The listing builds one solid part. Answer for the finished solid, in the listing's coordinates (mm). A direction names the side the tool comes from. Give positions to 0.01 mm unless a question says otherwise; leave off trailing zeros. Order: outer loops, then holes, each group sorted by start corner. A loop starts at its lowest first (then second) coordinate and runs counter-clockwise, first axis right, second up.
```python
from build123d import *

# Parameters (mm, degrees)
EXTRUDE_THIN1_DEPTH      = 100
F_4_0_4_DIAMETER_HOLE1_D = 4
FILLET3_R                = 5
FILLET2_R                = 1.5


with BuildPart() as part:
    # Sketch1 → Extrude-Thin1 (new body, symmetric)
    with BuildSketch(Plane(origin=(0, 0, 0), x_dir=(0, 0, -1), z_dir=(1, 0, 0))):
        Polygon((12.7, 40), (12.7, 0), (0, 0), (-12.7, 0), (-12.7, 20), (-17.7, 20), (-17.7, -5), (0, -5), (17.7, -5), (17.7, 40), align=None)
    extrude(amount=EXTRUDE_THIN1_DEPTH, both=True)

    # Ø4.0 (4) Diameter Hole1 (through all)
    with Locations(Plane(origin=(0, 13.65, 13.65), x_dir=(-1, 0, 0), z_dir=(0, 0.707106781, 0.707106781))):
        with Locations((80, -29.264527369), (-80, -29.264527369), (0, -29.264527369)):
            Hole(F_4_0_4_DIAMETER_HOLE1_D / 2)

    # Fillet3
    fillet3_edges = [part.edges().sort_by_distance(p)[0] for p in [
        (0, 0, -12.7),
    ]]
    fillet(fillet3_edges, radius=FILLET3_R)

    # Fillet2
    fillet2_edges = [part.edges().sort_by_distance(p)[0] for p in [
        (-100, 10, 12.7),
        (-100, 0, 2.5),
        (-100, 40, -15.2),
        (0, 20, 17.7),
        (0, 20, 12.7),
        (0, 0, 12.7),
        (0, 40, -12.7),
        (0, 40, -17.7),
        (100, 0, 2.5),
        (100, 10, 12.7),
        (100, 20, 15.2),
        (100, 7.5, 17.7),
        (-100, 22.5, -12.7),
        (100, 22.5, -12.7),
        (-100, 1.464466094, -11.235533906),
        (100, 1.464466094, -11.235533906),
        (100, 40, -15.2),
        (-100, 7.5, 17.7),
        (-100, 20, 15.2),
    ]]
    fillet(fillet2_edges, radius=FILLET2_R)


solid = part.part
```
1) Straight lines are drawn through the part: probe 1 along Z at (x, y) = (18, 14); probe 2 along Y at (x, z) = (8, 11); probe 3 along Y at (x, z) = (28.5, -14). For each, find the intervals that lie inside material, in ascending order.
Geometry says:
probe 1: z = -17.7 to -12.7, 12.7 to 17.7
probe 2: y = -5 to 0
probe 3: y = -5 to 39.99
2) Given P1, Ø5.5, axis at x = 19, z = 6, coming from the +Y side; P2, Ø8, axis at y = 3.5, z = -2, coming from the -X side; P3, Ø0.6, axis at x = -46.5, z = 15, coming from the +Y side; P4, Ø3, axis at y = 11, z = 10.5, coming from the +X side, each flat-ended and moving along its own axis, determine where each tip first touches the part or whether it passes through.
Geometry says:
P1: stops at y = 0
P2: stops at x = -99.62
P3: stops at y = 20
P4: passes through
3) A tool of negligible diameter and unlimited length cuts with its end or side. For faces 4 (the flat face through (1, 0, 2)), 5 (the cylindrical face through (-78.1, 25.7, -14.8)), from which of +Z, -Z, +X, -X, +Y, -Y can it reach the whole face along a straight path? Write none if from no direction.
Geometry says:
face 4: +X, -X, +Y
face 5: none
4) For a pull along Y with two mould halves and no side action, classify faces 1 (the cylindrical face through (81.9, 25.7, -14.8)), 2 (the flat face through (1, -5, 0)), 3 (the flat face through (1, 22, -12.7)) as +Y half, -Y half, draft (parallel to the pull), parting line (faces both ways), or undercut.
Geometry says:
face 1: undercut
face 2: -Y half
face 3: draft
5) Find section B-B (y = 26.5). Count the separate pieces of the cut face and the enclosed holes in it, then the cut area to 3 significant figures.
Geometry says:
separate pieces: 4
enclosed holes: 0
area: 949 mm2
6) Find section C-C (z = 4.5). Write down the section's boundary in (x, y), then the cut area to 3 significant figures.
Geometry says:
outline: (-100, -5) - (100, -5) - (100, -1.5) arc R1.5 ccw to (98.5, 0) - (-98.5, 0) arc R1.5 ccw to (-100, -1.5) - close
area: 999 mm2
7) Find section A-A (x = -26). Write down the section's boundary in (y, z).
Geometry says:
outline: (-5, -17.7) - (38.5, -17.7) arc R1.5 ccw to (40, -16.2) - (40, -14.2) arc R1.5 ccw to (38.5, -12.7) - (5, -12.7) arc R5 cw to (0, -7.7) - (0, 11.2) arc R1.5 cw to (1.5, 12.7) - (18.5, 12.7) arc R1.5 ccw to (20, 14.2) - (20, 16.2) arc R1.5 ccw to (18.5, 17.7) - (-5, 17.7) - close
